Build history of the part. All positions in model axes, mm. Face numbers are marked on the shaded views. A direction names the side the tool comes from. Give positions to 0.01 mm unless a question says otherwise; leave off trailing zeros. Order: outer loops, then holes, each group sorted by start corner. A loop starts at its lowest first (then second) coordinate and runs counter-clockwise, first axis right, second up. Notation, with made-up numbers: (-13.75, -13) -> (3.25, -13) arc R14 ccw to (3.25, 6) -> close; hole circle Ø3 at (14, -18). An arc over 180 degrees is marked (long way). Use a Markdown table: item, result. Add a question column.
Autodesk Fusion 360 part; units mm, degrees
sketch "Sketch1" plane through (0, 0, 0) normal (1, 0, 0) x (0, 0, -1)
  circle A0 centre (0, 0) radius 22.5
  dimension "d1" = 45
extrude "Extrude1" add sketch "Sketch1" along normal blind 3.2
sketch "Sketch2" plane through (3.2, 0, 0) normal (1, 0, 0) x (0, 0, -1)
  circle A0 centre (0, 0) radius 22.5
  circle A1 centre (0, 0) radius 20.5
  dimension "d4" = 41
extrude "Extrude2" add sketch "Sketch2" along normal blind 3.6 contours A1
sketch "Sketch3" plane through (6.8, 0, 0) normal (1, 0, 0) x (0, 0, -1)
  circle A0 centre (0, 0) radius 20.5
  circle A1 centre (0, 0) radius 22.5
  dimension "d7" = 45
extrude "Extrude3" add sketch "Sketch3" along normal blind 3.2 contours A0 | A1
fillet "Fillet1" radius 1.5 2 edges at (3.2, 7.4131, 19.1127) (6.8, -7.4131, 19.1127)
sketch "Sketch4" plane through (0, 0, 0) normal (-1, 0, 0) x (0, 0, 1)
  circle A0 centre (0, 0) radius 22.5
  circle A1 centre (0, 0) radius 28.9
  dimension "d11" = 57.8
extrude "Extrude4" add sketch "Sketch4" along normal blind 2.4 contours A0 | A1
sketch "Sketch5" plane through (0, 0, 0) normal (1, 0, 0) x (0, 0, -1)
  circle A0 centre (0, 0) radius 28.9
  circle A1 centre (0, 0) radius 22.5
  circle A2 centre (0, 0) radius 24.7
  dimension "d14" = 49.4
extrude "Extrude5" add sketch "Sketch5" along normal blind 1.8 contours A0
sketch "Sketch6" plane through (10, 0, 0) normal (1, 0, 0) x (0, 0, -1)
  circle A0 centre (0, 0) radius 22.5
  circle A1 centre (0, 0) radius 20.5
  circle A2 centre (0, 0) radius 18.1
  dimension "d17" = -2.4
extrude "Extrude6" cut sketch "Sketch6" against normal blind 10 contours A2
fillet "Fillet2" radius 1.2 1 edges at (10, -8.1363, 20.9774)
fillet "Fillet3" radius 1.6 1 edges at (-2.4, -10.4507, -26.9443)
fillet "Fillet4" radius 0.6 1 edges at (1.8, 8.9319, 23.0285)
equation "d4 = 44 mm - 3 mm"
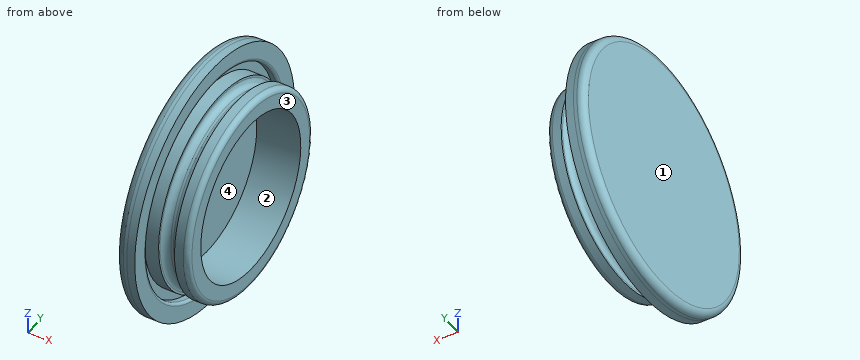
(1) Pin check, flat tips, straight feed: pin 1 Ø1.5 at (x, z) = (4.5, 15.5) entering from +Y; pin 2 Ø2 at (x, y) = (0, -1.5) entering from -Z; pin 3 Ø3 at (x, z) = (2, 14.5) entering from +Y. Stop position of each tip, or through.
(2) Wall check: probe 1 along Y at (x, z) = (0.8, 0); probe 2 along Z at (x, y) = (0.5, 8.5); probe 3 along X at (y, z) = (-8.5, 25). Give the ranges that are in metal, low to high.
(3) Band-saw the part on C-C on x = 7.5. Give the cut face in (y, z), plus the area to 3 significant figures.
(4) Tool access for the marked faces 3 and 4: list every direction of +Z, -Z, +X, -X, +Y, -Y with a clear straight run to the whole face (end or side of a thin tool).
(5) Mould opens along Y. For the marked faces 1 and 2 say: released by +Y, released by -Y, zero draft, split by the parting line, or undercut.
Response:
| question | item | result |
|---|---|---|
| 1 | pin 1 | stops at y = 14.3 |
| 1 | pin 2 | stops at z = -28.9 |
| 1 | pin 3 | stops at y = 25.8 |
| 2 | probe 1 | y = -28.9 to -24.7, -22.5 to -18.1, 18.1 to 22.5, 24.7 to 28.9 |
| 2 | probe 2 | z = -27.62 to -23.19, -20.83 to -15.98, 15.98 to 20.83, 23.19 to 27.62 |
| 2 | probe 3 | x = -2.4 to 1.8 |
| 3 | outline | circle Ø45 at (0, 0); hole circle Ø36.2 at (0, 0) |
| 3 | area | 561 mm² |
| 4 | face 3 | +Z, -Z, +X, +Y, -Y |
| 4 | face 4 | +X |
| 5 | face 1 | zero draft |
| 5 | face 2 | undercut |
